Could you check a few things on this model? Use its own coordinates, in mm. A direction names the side the tool comes from. Round coordinates to 2 decimals unless told otherwise and drop trailing zeros. Loops run counter-clockwise (first coordinate to the right, second up) from the corner with the lowest first, then second, coordinate; pieces in that order, holes last. Notation, with made-up numbers: M 27,-5 L 80,-5 A14 cw 80,20 Z; hole C 18,68.5 d9. An arc over 180 degrees is marked long. One line per item, written item: value. Start each with the question number.
Q1. Please list where these lines run through material, in increasing order: line 1 along X through (y, z) = (-8.5, 0); line 2 along X through (y, z) = (-5, 0).
Q2. Imagine slicing it at D-D (y = 11). Please give me the cut outline in (x, z), then the cut area to 3 significant figures.
Q3. Imagine slicing it at B-B (z = 3.75). Give the number of separate pieces and of enclosed holes in the cut face, then the cut area to 3 significant figures.
Q4. Which directions (+Z, -Z, +X, -X, +Y, -Y) give clear straight access to the entire face, cutting with the end or side of a thin tool? Please do faces 1 (the face through (-2.3, 6.65, 2.3)), 2 (the face through (-2.539, -18.885, 1.947)), 3 (the face through (-2.38, -7.76, 10.74)).
Q5. Thinking about a two-plate mould opening in Y: for faces 4 (the face through (-1.73, 10.13, 7.81)), 5 (the face through (-3, -12, 0)), which applies, released by +Y, released by -Y, zero draft, split by the parting line, or undercut?
Q6. Imagine slicing it at A-A (y = -3). Please give me the cut outline in (x, z).
Q7. I'm going to push flat-ended pins straight in: pin 1 Ø5 at (x, y) = (5, 8) entering from -Z; pin 2 Ø1 at (y, z) = (11, -5) entering from -X; pin 3 Ø5 at (x, y) = (-1, 10.5) entering from -Z. Where does each tip first touch, or does it pass through?
from build123d import *


with BuildPart() as part:
    # Sketch1 → Revolve1 (revolve)
    with BuildSketch(Plane.XY):
        Polygon((2.05, 21.35), (8, 21.35), (8, 17.65), (6, 17.65), (6, 11.65), (8, 11.65), (8, 8.65), (3, 8.65), (3, 6.65), (11, 6.65), (11, 5.85), (3, 5.85), (3, 3.85), (11, 3.85), (11, 3.05), (3, 3.05), (3, 1.05), (11, 1.05), (11, 0.25), (3, 0.25), (3, -1.75), (11, -1.75), (11, -2.55), (3, -2.55), (3, -4.55), (11, -4.55), (11, -5.35), (3, -5.35), (3, -7.35), (11, -7.35), (11, -8.15), (3, -8.15), (3, -10.15), (11, -10.15), (11, -10.95), (3, -10.95), (3, -12.95), (11, -12.95), (11, -13.75), (3.2, -13.75), (2.81308008, -13.75), (2.81308008, -16.35), (3.2, -16.35), (3.2, -21.35), (2.05, -21.35), align=None)
    revolve(axis=Axis((0, -21.35, 0), (0, 1, 0)))


solid = part.part
Report:
1. line 1: x = -3 to -2.05, 2.05 to 3
1. line 2: x = -11 to -2.05, 2.05 to 11
2. outline: C 0,0 d16; hole C 0,0 d4.1
2. area: 188 mm²
3. separate pieces: 9
3. enclosed holes: 0
3. area: 283 mm²
4. face 1: none
4. face 2: -Y
4. face 3: +Y, -Y
5. face 4: zero draft
5. face 5: undercut
6. outline: C 0,0 d6; hole C 0,0 d4.1
7. pin 1: stops at z = -10.61
7. pin 2: stops at x = -6.61
7. pin 3: stops at z = -8
